CAD build for the part. Positions are in the model's coordinates, mm. Give positions to 0.01 mm unless a question says otherwise; leave off trailing zeros. Loops run counter-clockwise (first coordinate to the right, second up) from the corner with the lowest first, then second, coordinate; pieces in that order, holes last. Notation, with made-up numbers: M 54,31.25 L 93,31.25 A9 ccw 93,37.25 Z; hole C 48.5,43 d2. An arc over 180 degrees is marked long. Answer as CSV lines item,"result".
```python
from build123d import *

# Parameters (mm, degrees)
SKETCH1_R           = 122.4
BOSS_EXTRUDE1_DEPTH = 6.35
SKETCH2_R           = 1.9939
CUT_EXTRUDE1_DEPTH  = 174.216172744
CIRPATTERN1_COUNT   = 4
SKETCH3_R           = 2.5
CUT_EXTRUDE3_DEPTH  = 174.216172744


with BuildPart() as part:
    # Sketch1 → Boss-Extrude1 (new body)
    with BuildSketch(Plane(origin=(0, 0, 0), x_dir=(1, 0, 0), z_dir=(0, 1, 0))):
        with Locations(Location((0, 0, 0), (0, 0, 270))):
            Circle(SKETCH1_R)
    extrude(amount=BOSS_EXTRUDE1_DEPTH)

    # Sketch2 → Cut-Extrude1 (cut, through all)
    with BuildSketch(Plane(origin=(0, 6.35, 0), x_dir=(1, 0, 0), z_dir=(0, 1, 0))):
        with Locations(Location((-19.05, -107.035541925, 0), (0, 0, 270))):
            Circle(SKETCH2_R)
        with Locations(Location((19.05, -107.035541925, 0), (0, 0, 270))):
            Circle(SKETCH2_R)
    cut_extrude1 = extrude(amount=-CUT_EXTRUDE1_DEPTH, mode=Mode.SUBTRACT)

    # CirPattern1: Cut-Extrude1 ×4 about axis
    cirpattern1_axis = Axis((0, 0, -0.056837174), (0, 1, 0))
    for i in range(1, CIRPATTERN1_COUNT):
        add(cut_extrude1.rotate(cirpattern1_axis, i * 360 / CIRPATTERN1_COUNT), mode=Mode.SUBTRACT)

    # Sketch3 → Cut-Extrude3 (cut, through all)
    with BuildSketch(Plane(origin=(0, 6.35, 0), x_dir=(1, 0, 0), z_dir=(0, 1, 0))):
        with Locations(Location((-74.054631747, 26.335816411, 0), (0, 0, 270))):
            Circle(SKETCH3_R)
        with Locations(Location((-39.054631747, 26.335816411, 0), (0, 0, 270))):
            Circle(SKETCH3_R)
        with Locations(Location((-16.113436886, -24.808749019, 0), (0, 0, 270))):
            Circle(SKETCH3_R)
        with Locations(Location((-74.054631747, -24.808749019, 0), (0, 0, 270))):
            Circle(SKETCH3_R)
    extrude(amount=-CUT_EXTRUDE3_DEPTH, mode=Mode.SUBTRACT)


solid = part.part
```
Q1. Wall check: line 1 (X direction, y = 2.5, z = -3); line 2 (Z direction, x = -25, y = 3); line 3 (X direction, y = 3, z = 75). Give the ranges that are in metal, low to high. Write a range as [from, to].
Solution:
line 1,"x = [-122.36, 122.36]"
line 2,"z = [-119.82, 119.82]"
line 3,"x = [-96.73, 96.73]"
Q2. Pin check, flat tips, straight feed: P1, Ø1.5, axis at y = 5, z = -28.5, coming from the +X side; P2, Ø1.5, axis at x = 31.5, y = 5.5, coming from the -Z side; P3, Ø3, axis at x = -26, y = 3, coming from the +Z side. Stop position of each tip, or through.
Solution:
P1,"stops at x = 119.21"
P2,"stops at z = -118.47"
P3,"stops at z = 119.92"
Q3. Cut at C-C (z = 88). Write the cut outline in (x, y).
Solution:
outline,"M -85.08,0 L 85.08,0 L 85.08,6.35 L -85.08,6.35 Z"
Q4. Cut at A-A (y = 2.25). Give the number of separate pieces and of enclosed holes in the cut face, and give its area (3 significant figures).
Solution:
separate pieces,"1"
enclosed holes,"12"
area,"46,900 mm²"
Q5. Cut at B-B (x = -79.5). Write the cut outline in (y, z).
Solution:
outline,"M 0,-93.07 L 6.35,-93.07 L 6.35,93.07 L 0,93.07 Z"
